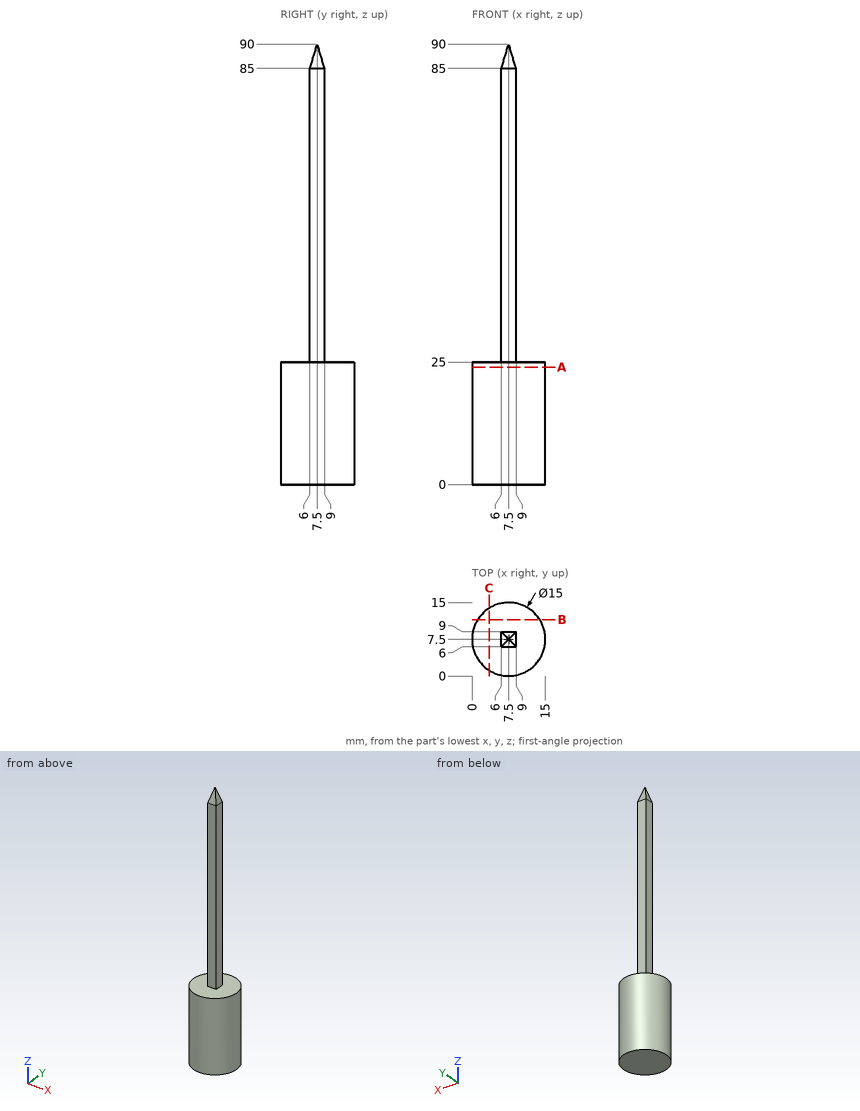
Verification items for this drawing (mm, ordinates from the low corner). Give positions to 0.01 mm unless a question says otherwise; leave off trailing zeros. Write each loop counter-clockwise with the first axis right and the second up, starting at its lowest first coordinate (ties: lowest second). Pieces come first, ordered by that corner, then holes.
1) Section check A-A, the plane z = 24. Record the boundary of the cut face in (x, y).
2) Section check B-B, the plane y = 11.5. Record the boundary of the cut face in (x, z).
3) Gauge pin test, flat ends, axial feed: pin 1 (8 mm diameter, centred on y = 8, z = 51, fed in from +X); pin 2 (0.9 mm diameter, centred on x = 7, z = 60.5, fed in from +Y); pin 3 (1.5 mm diameter, centred on y = 8, z = 43.5, fed in from -X). Record the tip position at first contact, or that the pin passes through.
4) Material ranges on L1, parallel to Z at x = 8.75, y = 12.25; L2, parallel to X at y = 6.5, z = 50, recorded low to high.
Computed:
1. outline: circle Ø15 at (7.5, 7.5)
2. outline: (1.16, 0) - (13.84, 0) - (13.84, 25) - (1.16, 25) - close
3. pin 1: stops at x = 9
3. pin 2: stops at y = 9
3. pin 3: stops at x = 6
4. L1: z = 0 to 25
4. L2: x = 6 to 9
